from build123d import *

# Parameters (mm, degrees)
SKETCH1_R           = 1.65
BOSS_EXTRUDE1_DEPTH = 5
CHAMFER1_SIZE       = 4
FILLET1_R           = 3


with BuildPart() as part:
    # Sketch1 → Boss-Extrude1 (new body)
    with BuildSketch(Plane(origin=(0, 0, 0), x_dir=(1, 0, 0), z_dir=(0, 1, 0))):
        Polygon((0, 0), (-52.5, 0), (-52.5, 29), (-39.5, 29), (-39.5, 15), (0, 15), align=None)
        with Locations(Location((-46, 25, 0), (0, 0, 270))):
            Circle(SKETCH1_R, mode=Mode.SUBTRACT)
    boss_extrude1 = extrude(amount=BOSS_EXTRUDE1_DEPTH)

    # Mirror1: Boss-Extrude1 across plane
    add(boss_extrude1.mirror(Plane(origin=(0, 0, 0), x_dir=(0, 0, 1), z_dir=(1, 0, 0))))

    # Chamfer1
    chamfer1_edges = [part.edges().sort_by_distance(p)[0] for p in [
        (-39.5, 2.5, -15),
        (39.5, 2.5, -15),
    ]]
    chamfer(chamfer1_edges, length=CHAMFER1_SIZE)

    # Fillet1
    fillet1_edges = [part.edges().sort_by_distance(p)[0] for p in [
        (-52.5, 2.5, -29),
        (52.5, 2.5, -29),
    ]]
    fillet(fillet1_edges, radius=FILLET1_R)


solid = part.part
Design review of the part built by this model. Coordinates are the model's own, in mm. A direction names the side the tool comes from. Give positions to 0.01 mm unless a question says otherwise; leave off trailing zeros. Order: outer loops, then holes, each group sorted by start corner. A loop starts at its lowest first (then second) coordinate and runs counter-clockwise, first axis right, second up.
1. Add section D-D, the plane x = -36.5. State the section outline as (y, z) points.
Solution:
outline: (0, -16) - (5, -16) - (5, 0) - (0, 0) - close
2. Add section B-B, the plane x = 46. State the section outline as (y, z) points, then the cut area to 4 significant figures.
Solution:
outline: (0, -29) - (5, -29) - (5, -26.65) - (0, -26.65) - close; (0, -23.35) - (5, -23.35) - (5, 0) - (0, 0) - close
area: 128.5 mm2
3. For pin 1 Ø1 at (x, y) = (25, 4) entering from -Z; pin 2 Ø2.5 at (x, z) = (-46, -25) entering from +Y, all flat-tipped, find the tip position at first contact; note any pin that passes through.
Solution:
pin 1: stops at z = -15
pin 2: passes through
4. Add section A-A, the plane y = 4. State the section outline as (x, z) points.
Solution:
outline: (-52.5, -26) arc R3 ccw to (-49.5, -29) - (-39.5, -29) - (-39.5, -19) - (-35.5, -15) - (35.5, -15) - (39.5, -19) - (39.5, -29) - (49.5, -29) arc R3 ccw to (52.5, -26) - (52.5, 0) - (-52.5, 0) - close; hole circle Ø3.3 at (-46, -25); hole circle Ø3.3 at (46, -25)
5. Mouldability with a two-part tool opening along X and no side actions: class faces 3 (the flat face through (-39.5, 2, -24)), 4 (the flat face through (39.5, 2, -24)), 5 (the flat face through (-1, 2, 0)), 6 (the flat face through (-52.5, 2, -13)) as +X half, -X half, draft (parallel to the pull), parting line (faces both ways), or undercut.
Solution:
face 3: undercut
face 4: undercut
face 5: draft
face 6: -X half
6. Tool access review of faces 1 (the flat face through (-1, 0, -11)), 2 (the flat face through (0, 2, -15)): name each direction out of +Z, -Z, +X, -X, +Y, -Y from which nothing blocks a thin tool from reaching the whole face with its end or side.
Solution:
face 1: +Z, -Z, +X, -X, -Y
face 2: -Z, +Y, -Y
7. Add section C-C, the plane z = -25. State the section outline as (x, y) points, then the cut area to 3 significant figures.
Solution:
outline: (-52.5, 0) - (-47.65, 0) - (-47.65, 5) - (-52.5, 5) - close; (-44.35, 0) - (-39.5, 0) - (-39.5, 5) - (-44.35, 5) - close; (39.5, 0) - (44.35, 0) - (44.35, 5) - (39.5, 5) - close; (47.65, 0) - (52.5, 0) - (52.5, 5) - (47.65, 5) - close
area: 97.0 mm2
8. To check wall thickness, follow L1, parallel to X at y = 2.75, z = -25; L2, parallel to X at y = 4.7, z = -21; L3, parallel to Z at x = 46, y = 1.8. State the ranges of each line that lie inside material, in increasing order.
Solution:
L1: x = -52.5 to -47.65, -44.35 to -39.5, 39.5 to 44.35, 47.65 to 52.5
L2: x = -52.5 to -39.5, 39.5 to 52.5
L3: z = -29 to -26.65, -23.35 to 0
